```python
from build123d import *

# Parameters (mm, degrees)
SKETCH_1_W      = 54
SKETCH_1_H      = 38.5
SKETCH_1_R      = 1.5
SKETCH_1_R_2    = 3
EXTRUDE_1_DEPTH = 2.4
FILLET_1_R      = 4


with BuildPart() as part:
    # 草圖1 → 填料-伸長1 (new body)
    with BuildSketch(Plane(origin=(0, 0, 0), x_dir=(1, 0, 0), z_dir=(0, 1, 0))):
        with Locations((0, 14.25)):
            Rectangle(SKETCH_1_W, SKETCH_1_H)
        with Locations((-24, 0)):
            Circle(SKETCH_1_R, mode=Mode.SUBTRACT)
        with Locations((24, 0)):
            Circle(SKETCH_1_R, mode=Mode.SUBTRACT)
        with Locations((-10.5, 28.5)):
            Circle(SKETCH_1_R_2, mode=Mode.SUBTRACT)
        with Locations((10.5, 28.5)):
            Circle(SKETCH_1_R_2, mode=Mode.SUBTRACT)
        with Locations((-10.5, 0)):
            Circle(SKETCH_1_R_2, mode=Mode.SUBTRACT)
        with Locations((10.5, 0)):
            Circle(SKETCH_1_R_2, mode=Mode.SUBTRACT)
        with Locations((24, 20)):
            Circle(SKETCH_1_R, mode=Mode.SUBTRACT)
        with Locations((-24, 20)):
            Circle(SKETCH_1_R, mode=Mode.SUBTRACT)
    extrude(amount=EXTRUDE_1_DEPTH)

    # 圓角1
    fillet_1_edges = [part.edges().sort_by_distance(p)[0] for p in [
        (27, 1.2, 5),
        (-27, 1.2, 5),
        (-27, 1.2, -33.5),
        (27, 1.2, -33.5),
    ]]
    fillet(fillet_1_edges, radius=FILLET_1_R)


solid = part.part
```
Check sheet for the modelled part. Datum: model origin and axes. Units: mm. Coordinates: 2 decimals unless noted, no trailing zeros. Write each loop counter-clockwise with the first axis right and the second up, starting at its lowest first coordinate (ties: lowest second). Pieces come first, ordered by that corner, then holes. Notation, with made-up numbers: (44.25, -22.5) -> (50.25, -22.5) arc R18 ccw to (50.25, -1.5) -> close; hole circle Ø10 at (77.5, 37). An arc over 180 degrees is marked (long way). Use a Markdown table: item, result.
1. Sectioned sample at A-A (z = -20). Enter the section's corners in (x, y).
Reported:
| item | result |
|---|---|
| outline | (-27, 0) -> (-25.5, 0) -> (-25.5, 2.4) -> (-27, 2.4) -> close; (-22.5, 0) -> (22.5, 0) -> (22.5, 2.4) -> (-22.5, 2.4) -> close; (25.5, 0) -> (27, 0) -> (27, 2.4) -> (25.5, 2.4) -> close |
2. Scan lines: line 1 along X through (y, z) = (0.85, 0); line 2 along Z through (x, y) = (-10.5, 1.7); line 3 along X through (y, z) = (1.7, -20). Record each from-to range of solid material in increasing order.
Reported:
| item | result |
|---|---|
| line 1 | x = -27 to -25.5, -22.5 to -13.5, -7.5 to 7.5, 13.5 to 22.5, 25.5 to 27 |
| line 2 | z = -33.5 to -31.5, -25.5 to -3, 3 to 5 |
| line 3 | x = -27 to -25.5, -22.5 to 22.5, 25.5 to 27 |
3. Sectioned sample at C-C (y = 1.25). Give the number of separate pieces and of enclosed holes in the cut face, plus the area to 3 significant figures.
Reported:
| item | result |
|---|---|
| separate pieces | 1 |
| enclosed holes | 8 |
| area | 1,920 mm2 |
4. Go/stop test with flat-tipped pins: pin 1 Ø12 at (x, z) = (12.5, -12) entering from -Y; pin 2 Ø2.5 at (x, z) = (24, -20) entering from +Y. Record where each tip stops, or that it passes through.
Reported:
| item | result |
|---|---|
| pin 1 | stops at y = 0 |
| pin 2 | passes through |
5. Release check for a two-part mould opening along X. For faces 1 (the flat face through (0, 1, 5)), 2 (the cylindrical face through (-25.5, 1.18, -0.07)), 3 (the cylindrical face through (25.797, 1.217, -32.359)) record: pulls with the +X half, pulls with the -X half, needs draft (parallel to the pull), parting line crosses it, or undercut.
Reported:
| item | result |
|---|---|
| face 1 | needs draft |
| face 2 | undercut |
| face 3 | pulls with the +X half |
6. Sectioned sample at B-B (x = 10.5). Enter the section's corners in (y, z).
Reported:
| item | result |
|---|---|
| outline | (0, -33.5) -> (2.4, -33.5) -> (2.4, -31.5) -> (0, -31.5) -> close; (0, -25.5) -> (2.4, -25.5) -> (2.4, -3) -> (0, -3) -> close; (0, 3) -> (2.4, 3) -> (2.4, 5) -> (0, 5) -> close |
